Could you check a few things on this model? Use its own coordinates, in mm. A direction names the side the tool comes from. Round coordinates to 2 decimals unless told otherwise and drop trailing zeros. Write each loop counter-clockwise with the first axis right and the second up, starting at its lowest first coordinate (ties: lowest second). Pieces come first, ordered by that corner, then holes. Notation, with made-up numbers: (56.25, -3) -> (82.25, -3) arc R32 cw to (82.25, 31) -> close; hole circle Ø4 at (-34.5, -18). An arc over 180 degrees is marked (long way). Answer in a Markdown table with one row per item.
Autodesk Inventor part; units mm, degrees
ref_plane "Work Plane1" through (15, 0, 0) normal (1, 0, 0) x (0, 0, -1)
ref_plane "YZ Plane" through (0, 0, 0) normal (1, 0, 0) x (0, 1, 0)
ref_plane "XZ Plane" through (0, 0, 0) normal (0, 1, 0) x (-1, 0, 0)
sketch "Sketch1" plane through (0, 0, 0) normal (1, 0, 0) x (0, 1, 0)
  circle A0 centre (0, 0) radius 2.5
  line L0 (-10, 10) -> (10, 10)
  line L1 (10, 10) -> (10, -10)
  line L2 (10, -10) -> (-10, -10)
  line L3 (-10, -10) -> (-10, 10)
  line L4 (-10, 10) -> (10, -10) construction
  line L5 (10, 10) -> (-10, -10) construction
  dimension "d0" = 5
  dimension "d1" = 20
  dimension "d2" = 20
extrude "Extrusion1" add sketch "Sketch1" along normal blind 20
ref_plane "Work Plane1" through (15, 0, 0) normal (1, 0, 0) x (0, 0, -1)
sketch "Sketch2" plane through (15, 0, 0) normal (1, 0, 0) x (0, 0, -1)
  line L0 (10, -10) -> (10, 10)
  line L1 (-10, -10) -> (10, -10)
  line L2 (10, -10) -> (10, 10)
  line L3 (10, 10) -> (-10, 10)
  line L4 (-10, 10) -> (-10, -10)
  line L5 (-10, -10) -> (10, 10) construction
  line L6 (10, -10) -> (-10, 10) construction
  line L7 (-7.5, -7.5) -> (7.5, -7.5)
  line L8 (7.5, -7.5) -> (7.5, 7.5)
  line L9 (7.5, 7.5) -> (-7.5, 7.5)
  line L10 (-7.5, 7.5) -> (-7.5, -7.5)
  line L11 (-7.5, -7.5) -> (7.5, 7.5) construction
  line L12 (7.5, -7.5) -> (-7.5, 7.5) construction
  point P0 (0, 0)
  dimension "d6" = 15
  dimension "d7" = 15
extrude "Extrusion2" cut sketch "Sketch2" against normal blind 10
chamfer "Chamfer1" distance 4 angle 45 4 edges at (17.5, 10, 10) (17.5, 10, -10) (17.5, -10, -10) (17.5, -10, 10)
properties part number "Servo Motor"
1) For pin 1 (8 mm diameter, centred on y = 0, z = 0, fed in from -X); pin 2 (5 mm diameter, centred on x = 11, z = 3.5, fed in from +Y); pin 3 (8 mm diameter, centred on x = 10, z = 3, fed in from -Y); pin 4 (5 mm diameter, centred on x = 10, y = 1.5, fed in from -Z), each with a flat end and sliding along its axis, tell me the tip position at first contact or that it passes through.
Findings:
| item | result |
|---|---|
| pin 1 | stops at x = 0 |
| pin 2 | stops at y = 7.5 |
| pin 3 | stops at y = -7.5 |
| pin 4 | stops at z = -7.5 |
2) Imagine slicing it at A-A, the plane y = 0. Please give me the cut outline in (x, z), plus the area to 3 significant figures.
Findings:
| item | result |
|---|---|
| outline | (0, -10) -> (5, -10) -> (5, -7.5) -> (15, -7.5) -> (15, -10) -> (20, -10) -> (20, -2.5) -> (0, -2.5) -> close; (0, 2.5) -> (20, 2.5) -> (20, 10) -> (15, 10) -> (15, 7.5) -> (5, 7.5) -> (5, 10) -> (0, 10) -> close |
| area | 250 mm^2 |
3) Imagine slicing it at D-D, the plane y = -6.5. Please give me the cut outline in (x, z).
Findings:
| item | result |
|---|---|
| outline | (0, -10) -> (5, -10) -> (5, -7.5) -> (15, -7.5) -> (15, -9.5) -> (20, -9.5) -> (20, 9.5) -> (15, 9.5) -> (15, 7.5) -> (5, 7.5) -> (5, 10) -> (0, 10) -> close |
4) For faces 4 (the face through (10, 0, -7.5)), 5 (the face through (17, 8, -8)), 6 (the face through (17, 8, 8)), 7 (the face through (15, 8, 0)), which set-ups out of +Z, -Z, +X, -X, +Y, -Y let a thin tool reach every point of the face, with its end or its side?
Findings:
| item | result |
|---|---|
| face 4 | -Z, +Y, -Y |
| face 5 | -Z, +X, +Y |
| face 6 | +Z, +X, +Y |
| face 7 | none |
5) Please list where these lines run through material, in increasing order: line 1 (X direction, y = -3.25, z = -8); line 2 (Z direction, x = 7, y = 0); line 3 (Y direction, x = 12, z = 3).
Findings:
| item | result |
|---|---|
| line 1 | x = 0 to 5, 15 to 20 |
| line 2 | z = -7.5 to -2.5, 2.5 to 7.5 |
| line 3 | y = -7.5 to 7.5 |
6) Thinking about a two-plate mould opening in X: for faces 1 (the face through (20, 2, 2)), 2 (the face through (17, 0, 10)), 3 (the face through (5, 0, 9)), which applies, +X half, -X half, draft (parallel to the pull), parting line (faces both ways), or undercut?
Findings:
| item | result |
|---|---|
| face 1 | +X half |
| face 2 | draft |
| face 3 | undercut |
7) Imagine slicing it at C-C, the plane x = 19. Please give me the cut outline in (y, z), plus the area to 3 significant figures.
Findings:
| item | result |
|---|---|
| outline | (-10, -6) -> (-6, -10) -> (6, -10) -> (10, -6) -> (10, 6) -> (6, 10) -> (-6, 10) -> (-10, 6) -> close; hole circle Ø5 at (0, 0) |
| area | 348 mm^2 |
